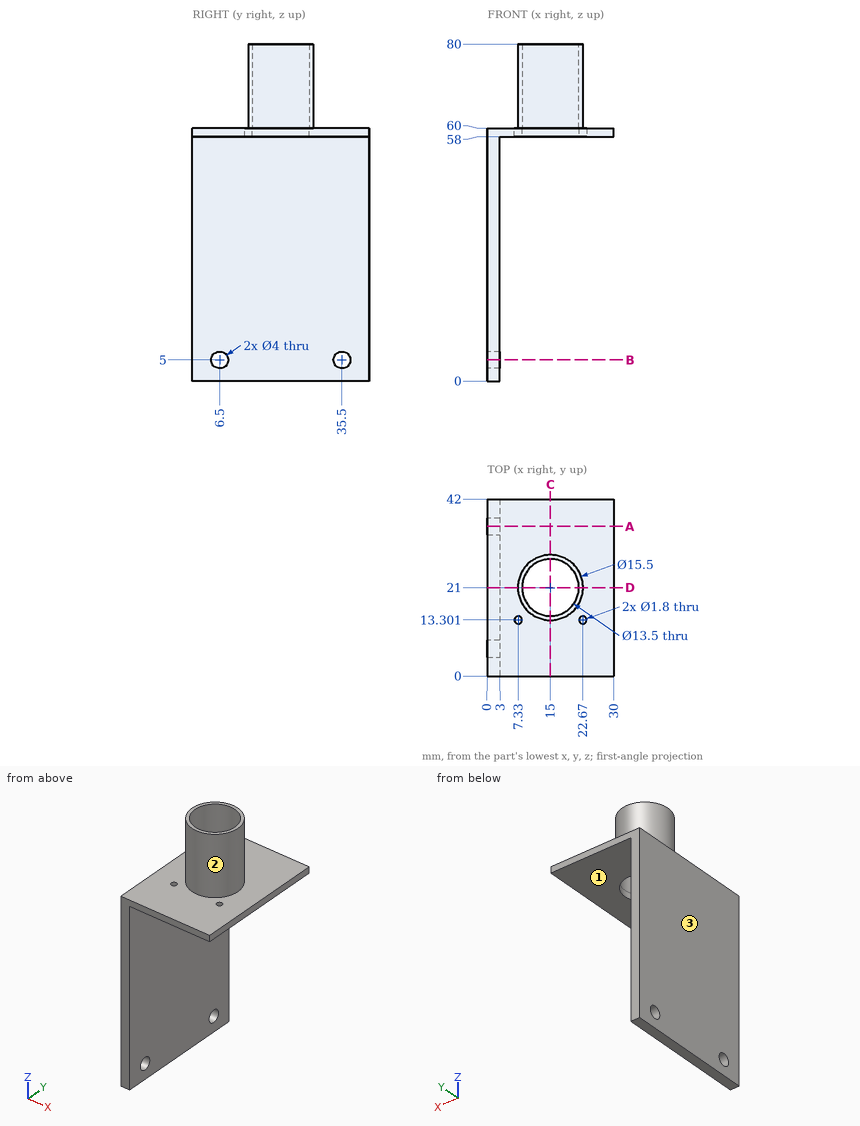
Can you work these out from the drawing? Everything is in mm from the part's minimum corner. A direction names the side the tool comes from. Give positions to 0.01 mm unless a question says otherwise; leave off trailing zeros. Order: outer loops, then holes, each group sorted by start corner. A loop starts at its lowest first (then second) coordinate and runs counter-clockwise, first axis right, second up. Notation, with made-up numbers: M 28,-5.5 L 42,-5.5 A22 cw 42,5.5 Z; hole C 9,-28 d4. An arc over 180 degrees is marked long. Use a Markdown table: item, result. Add a question column.
Item 1: If I drill on L1, parallel to Y at x = 22.67, z = 59.05; L2, parallel to Z at x = 1.2, y = 35.5; L3, parallel to Z at x = 3.5, y = 20, over which ranges is the centre line in solid material (lowest first)? Write a range as [from, to].
Item 2: Suppose I cut it at C-C (x = 15). List the corners of the cut face in (y, z) for me.
Item 3: Suppose I cut it at B-B (z = 5). List the corners of the cut face in (x, y) for me.
Item 4: Suppose I cut it at A-A (y = 35.5). List the corners of the cut face in (x, z) for me, then the cut area to 3 significant figures.
Item 5: For the marked faces 1, 2 and 3, which set-ups out of +Z, -Z, +X, -X, +Y, -Y let a thin tool reach every point of the face, with its end or its side?
Item 6: Suppose I cut it at D-D (y = 21). List the corners of the cut face in (x, z) for me, then the cut area to 3 significant figures.
Item 7: Will these pins go through, and if not, where does the flat tip stop? pin 1 (1.6 mm diameter, centred on x = 22.67, y = 13.3, fed in from -Z); pin 2 (5 mm diameter, centred on x = 24.5, z = 69.5, fed in from -Y); pin 3 (1 mm diameter, centred on x = 24.5, y = 36.5, fed in from -Z); pin 4 (3 mm diameter, centred on y = 12.5, z = 13.5, fed in from +X).
Answer sheet:
| question | item | result |
|---|---|---|
| 1 | L1 | y = [0, 12.4], [14.2, 42] |
| 1 | L2 | z = [0, 3], [7, 60] |
| 1 | L3 | z = [58, 60] |
| 2 | outline | M 0,58 L 14.25,58 L 14.25,80 L 13.25,80 L 13.25,60 L 0,60 Z; M 27.75,58 L 42,58 L 42,60 L 28.75,60 L 28.75,80 L 27.75,80 Z |
| 3 | outline | M 0,0 L 3,0 L 3,4.5 L 0,4.5 Z; M 0,8.5 L 3,8.5 L 3,33.5 L 0,33.5 Z; M 0,37.5 L 3,37.5 L 3,42 L 0,42 Z |
| 4 | outline | M 0,0 L 3,0 L 3,3 L 0,3 Z; M 0,7 L 3,7 L 3,58 L 30,58 L 30,60 L 0,60 Z |
| 4 | area | 222 mm² |
| 5 | face 1 | -Z, +X, +Y, -Y |
| 5 | face 2 | +Z |
| 5 | face 3 | +Z, -Z, -X, +Y, -Y |
| 6 | outline | M 0,0 L 3,0 L 3,58 L 8.25,58 L 8.25,80 L 7.25,80 L 7.25,60 L 0,60 Z; M 21.75,58 L 30,58 L 30,60 L 22.75,60 L 22.75,80 L 21.75,80 Z |
| 6 | area | 247 mm² |
| 7 | pin 1 | passes through |
| 7 | pin 2 | stops at y = 17.67 |
| 7 | pin 3 | stops at z = 58 |
| 7 | pin 4 | stops at x = 3 |
